```python
from build123d import *

# Parameters (mm, degrees)
RESSALTO_EXTRUS_O1_DEPTH   = 23.85
CHANFRO1_SIZE              = 7
CORTE_EXTRUS_O1_DEPTH      = 65.048254304
CORTE_EXTRUS_O1_DEPTH_BACK = 65.048254304
ESBO_O2_R                  = 5.25


with BuildPart() as part:
    # Esboço1 → Ressalto-extrusão1 (new body)
    with BuildSketch(Plane.XY):
        Polygon((-57.364870118, 0), (-31.364870118, 0), (31.635129882, 14.544696041), (57.635129882, 14.544696041), (57.635129882, 13.344696041), (31.635129882, 13.344696041), (-31.364870118, -1.2), (-57.364870118, -1.2), align=None)
    extrude(amount=RESSALTO_EXTRUS_O1_DEPTH)

    # Chanfro1
    chanfro1_edges = [part.edges().sort_by_distance(p)[0] for p in [
        (57.635129882, 13.944696041, 23.85),
        (-57.364870118, -0.6, 23.85),
    ]]
    chamfer(chanfro1_edges, length=CHANFRO1_SIZE)

    # Esboço2 → Corte-extrusão1 (cut, two sides: drawn at the far end of the back side and taken through both)
    with BuildSketch(Plane(origin=(0, 0, 0), x_dir=(1, 0, 0), z_dir=(0, 1, 0)).offset(-CORTE_EXTRUS_O1_DEPTH_BACK)):
        with Locations(Location((-44.914870118, -11.925, 0), (0, 0, 270))):
            Circle(ESBO_O2_R)
        with Locations(Location((45.185129882, -11.925, 0), (0, 0, 180))):
            Circle(ESBO_O2_R)
    extrude(amount=CORTE_EXTRUS_O1_DEPTH + CORTE_EXTRUS_O1_DEPTH_BACK, mode=Mode.SUBTRACT)


solid = part.part
```
Model file for the job. Use its own axes, mm. A direction names the side the tool comes from. Give positions to 0.01 mm unless a question says otherwise; leave off trailing zeros. Loops run counter-clockwise (first coordinate to the right, second up) from the corner with the lowest first, then second, coordinate; pieces in that order, holes last. Notation, with made-up numbers: (-27.5, 72.25) - (-19.5, 72.25) arc R22 ccw to (-19.5, 93.25) - close; hole circle Ø11 at (64.25, 69). An arc over 180 degrees is marked (long way). One line per item, written item: value. Start each with the question number.
1. Slice it at C-C (z = 5). List the corners of the cut face in (x, y), plus the area to 3 significant figures.
2. Pull direction Z, two halves, no side cores. Call faces 1 (the flat face through (54.086, 13.953, 20.399)), 2 (the cylindrical face through (-49.57, -0.61, 14.35)), 3 (the flat face through (45, 13.345, 6)): pulls with the +Z half, pulls with the -Z half, needs draft (parallel to the pull), parting line crosses it, or undercut.
3. Pin check, flat tips, straight feed: pin 1 (6.5 mm diameter, centred on x = -44.91, z = 11.92, fed in from +Y); pin 2 (4 mm diameter, centred on x = 33.5, z = 3, fed in from -Y); pin 3 (5 mm diameter, centred on x = 15, z = 12, fed in from +Y); pin 4 (10 mm diameter, centred on x = -2.5, z = 5, fed in from +Y). Stop position of each tip, or through.
4. Probe L1, parallel to Y at x = -36, z = 4.75; L2, parallel to Y at x = 39.5, z = 21.5. List the from-to ranges inside material, lowest first. Write a range as from..to.
5. Slice it at D-D (y = 8). List the corners of the cut face in (x, z), plus the area to 3 significant figures.
6. Slice it at B-B (x = 46.5). List the corners of the cut face in (y, z).
7. Which spindle directions (+Z, -Z, +X, -X, +Y, -Y) get a long thin tool onto all of the face, cutting with end or side? Do faces 4 (the flat face through (0, 7, 23.85)), 5 (the flat face through (-45, 0, 6)). Say none if no direction does.
8. Slice it at A-A (z = 14). List the corners of the cut face in (x, y).
Solution:
1. outline: (-57.36, -1.2) - (-31.36, -1.2) - (31.64, 13.34) - (57.64, 13.34) - (57.64, 14.54) - (31.64, 14.54) - (-31.36, 0) - (-57.36, 0) - close
1. area: 138 mm^2
2. face 1: pulls with the +Z half
2. face 2: undercut
2. face 3: needs draft
3. pin 1: passes through
3. pin 2: stops at y = 13.31
3. pin 3: stops at y = 11.28
3. pin 4: stops at y = 7.82
4. L1: y = -1.2..0
4. L2: y = 13.34..14.54
5. outline: (3.29, 0) - (8.48, 0) - (8.48, 23.85) - (3.29, 23.85) - close
5. area: 124 mm^2
6. outline: (13.34, 0) - (14.54, 0) - (14.54, 6.84) - (13.34, 6.84) - close; (13.34, 17.01) - (14.54, 17.01) - (14.54, 23.85) - (13.34, 23.85) - close
7. face 4: +Z, +X, -X, +Y, -Y
7. face 5: +Z, -Z, -X, +Y
8. outline: (-57.36, -1.2) - (-49.74, -1.2) - (-49.74, 0) - (-57.36, 0) - close; (-40.09, -1.2) - (-31.36, -1.2) - (31.64, 13.34) - (40.36, 13.34) - (40.36, 14.54) - (31.64, 14.54) - (-31.36, 0) - (-40.09, 0) - close; (50.01, 13.34) - (57.64, 13.34) - (57.64, 14.54) - (50.01, 14.54) - close
